Autodesk Inventor part; units mm, degrees
ref_plane "YZ Plane" through (0, 0, 0) normal (1, 0, 0) x (0, 1, 0)
ref_plane "XZ Plane" through (0, 0, 0) normal (0, 1, 0) x (-1, 0, 0)
ref_plane "XY Plane" through (0, 0, 0) normal (0, 0, 1) x (1, 0, 0)
sketch "Sketch1" plane through (0, 0, 0) normal (0, 0, 1) x (1, 0, 0)
  circle A0 centre (0, 0) radius 10
  circle A1 centre (0, 0) radius 30
  circle A2 centre (0, 15) radius 1.25
  circle A3 centre (-12.9904, -7.5) radius 1.25
  circle A4 centre (12.9904, -7.5) radius 1.25
  dimension "d0" = 20
  dimension "d1" = 60
  dimension "d3" = 2.5
  dimension "d6" = 360
extrude "Extrusion1" add sketch "Sketch1" along normal blind 5
sketch "Sketch5" plane through (0, 0, 5) normal (0, 0, 1) x (1, 0, 0)
  circle A0 centre (0, 0) radius 25 construction
  circle A1 centre (25, 0) radius 2.25
  dimension "d40" = 50
  dimension "d41" = 4.5
hole "Hole1" at (25, 0, 5) direction (0, 0, -1) diameter 4.5 end through all counterbore diameter 8 counterbore depth 2
pattern_circular "Circular Pattern2" count 3 over 360 about axis through (0, 0, 0) along (0, 0, 1) of "Hole1"
sketch "Sketch4" plane through (0, 0, 5) normal (0, 0, 1) x (1, 0, 0)
  circle A0 centre (0, 0) radius 10
  circle A1 centre (0, 0) radius 11
  dimension "d34" = 1
extrude "Extrusion8" cut sketch "Sketch4" against normal blind 10
properties part number "Encoder Mount Front" material "ABS Plastic"
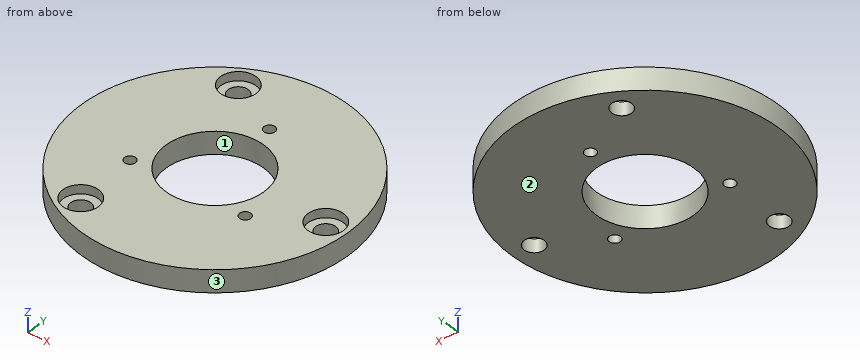
Check sheet for the modelled part. Datum: model origin and axes. Units: mm. Face numbers are marked on the shaded views. Round coordinates to 2 decimals unless told otherwise and drop trailing zeros. Loops run counter-clockwise (first coordinate to the right, second up) from the corner with the lowest first, then second, coordinate; pieces in that order, holes last. Notation, with made-up numbers: (-11.75, 43.25) - (-6.75, 43.25) arc R19 ccw to (-6.75, 68.25) - close; hole circle Ø5 at (66, 3.25). An arc over 180 degrees is marked (long way). Write item = value, one per line. Start each with the question number.
Q1. Thickness scan on L1, parallel to Y at x = 0, z = 2.55; L2, parallel to X at y = -2, z = 1.4; L3, parallel to Y at x = 4, z = 3.8. Record the ranges inside material, lowest first.
Q2. Section check A-A (y = 0). Record the boundary of the cut face in (x, z), plus the area to 4 significant figures.
Q3. Section check D-D (y = -7.5). Record the boundary of the cut face in (x, z), plus the area to 3 significant figures.
Q4. Depth check by flat-ended pin: P1, Ø3.5, axis at x = -12.5, y = -21.65, coming from the +Z side; P2, Ø2, axis at x = 7, z = 4.5, coming from the +Y side; P3, Ø2, axis at y = -14.5, z = 2, coming from the -X side; P4, Ø4, axis at x = 25, y = -0.5, coming from the +Z side. Enter the tip coordinate at first touch or a pass-through.
Q5. Release check for a two-part mould opening along X. For the marked faces 1, 2 and 3 record: pulls with the +X half, pulls with the -X half, needs draft (parallel to the pull), parting line crosses it, or undercut.
Q6. Section check B-B (x = 0). Record the boundary of the cut face in (y, z), plus the area to 4 significant figures.
Q7. Section check C-C (x = 25). Record the boundary of the cut face in (y, z).
Derived:
q1.L1 = -30 to -11, 11 to 13.75, 16.25 to 30
q1.L2 = -29.93 to -10.82, 10.82 to 23.97, 26.03 to 29.93
q1.L3 = -29.73 to -10.25, 10.25 to 29.73
q2.outline = (-30, 0) - (-11, 0) - (-11, 5) - (-30, 5) - close; (11, 0) - (22.75, 0) - (22.75, 3) - (21, 3) - (21, 5) - (11, 5) - close; (27.25, 0) - (30, 0) - (30, 5) - (29, 5) - (29, 3) - (27.25, 3) - close
q2.area = 160.5 mm^2
q3.outline = (-29.05, 0) - (-14.24, 0) - (-14.24, 5) - (-29.05, 5) - close; (-11.74, 0) - (-8.05, 0) - (-8.05, 5) - (-11.74, 5) - close; (8.05, 0) - (11.74, 0) - (11.74, 5) - (8.05, 5) - close; (14.24, 0) - (29.05, 0) - (29.05, 5) - (14.24, 5) - close
q3.area = 185 mm^2
q4.P1 = through
q4.P2 = 29.39
q4.P3 = -26.79
q4.P4 = 3
q5.face_1 = undercut
q5.face_2 = needs draft
q5.face_3 = parting line crosses it
q6.outline = (-30, 0) - (-11, 0) - (-11, 5) - (-30, 5) - close; (11, 0) - (13.75, 0) - (13.75, 5) - (11, 5) - close; (16.25, 0) - (30, 0) - (30, 5) - (16.25, 5) - close
q6.area = 177.5 mm^2
q7.outline = (-16.58, 0) - (-2.25, 0) - (-2.25, 3) - (-4, 3) - (-4, 5) - (-16.58, 5) - close; (2.25, 0) - (16.58, 0) - (16.58, 5) - (4, 5) - (4, 3) - (2.25, 3) - close
